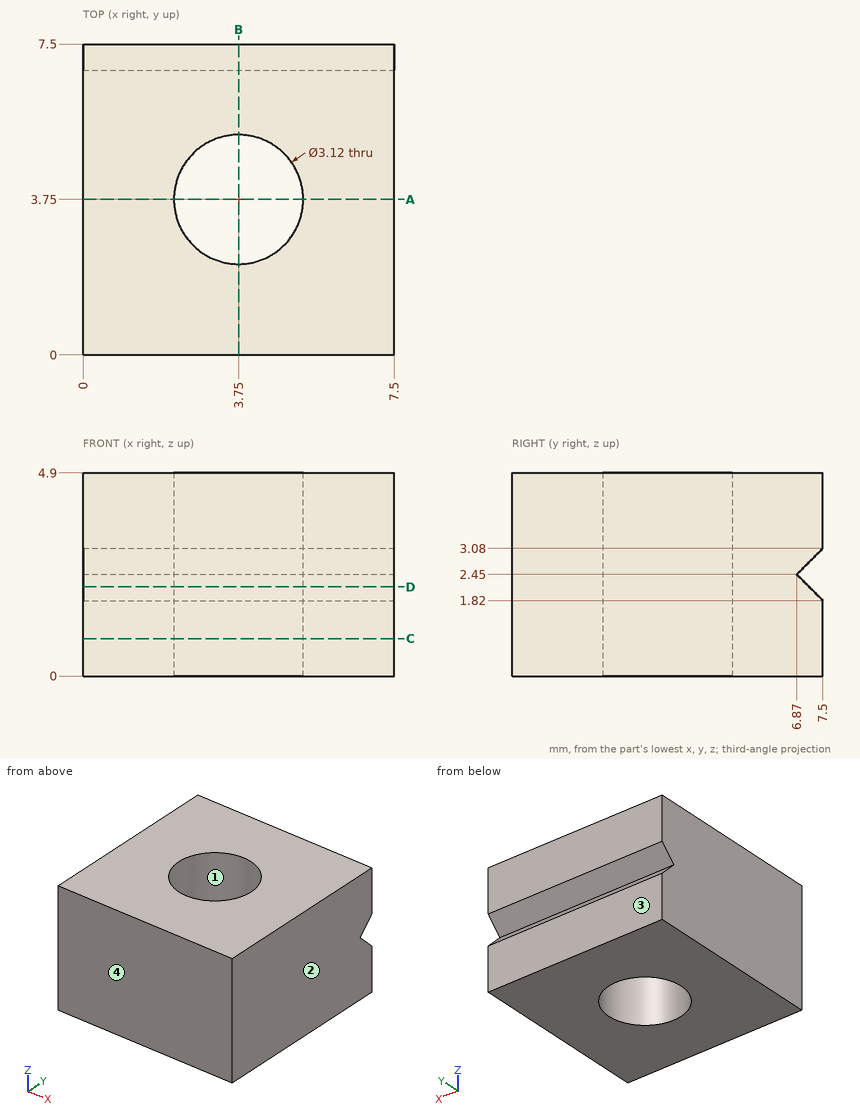
The figure shows three views and two pictorial views of one solid part (mm, origin at its lowest corner). Answer the questions. Coordinates: 2 decimals unless noted, no trailing zeros. Loops run counter-clockwise (first coordinate to the right, second up) from the corner with the lowest first, then second, coordinate; pieces in that order, holes last. Notation, with made-up numbers: (19.25, -8.5) -> (39.25, -8.5) arc R31 ccw to (39.25, 25.5) -> close; hole circle Ø2 at (63.5, 77.25). An arc over 180 degrees is marked (long way). Use one line per item in the form item = value. Start each with the question number.
Item 1: The part is cut by section C-C on z = 0.9. Determine the outline of the cut face in (x, y).
Item 2: The part is cut by section B-B on x = 3.75. Determine the outline of the cut face in (y, z).
Item 3: Consider L1, parallel to Y at x = 3.75, z = 1.3; L2, parallel to X at y = 3, z = 0.55; L3, parallel to Z at x = 4.25, y = 7.25. Determine where each line is inside the solid, lowest interval first. Write a range as [from, to].
Item 4: The part is cut by section D-D on z = 2.15. Determine the outline of the cut face in (x, y).
Item 5: The part is cut by section A-A on y = 3.75. Determine the outline of the cut face in (x, z).
Item 6: The mould has two halves that part along Y. Classify the marked faces 1, 2, 3 and 4: released by +Y, released by -Y, zero draft, split by the parting line, or undercut.
Answer key:
q1.outline = (0, 0) -> (7.5, 0) -> (7.5, 7.5) -> (0, 7.5) -> close; hole circle Ø3.12 at (3.75, 3.75)
q2.outline = (0, 0) -> (2.19, 0) -> (2.19, 4.9) -> (0, 4.9) -> close; (5.31, 0) -> (7.5, 0) -> (7.5, 1.82) -> (6.87, 2.45) -> (7.5, 3.08) -> (7.5, 4.9) -> (5.31, 4.9) -> close
q3.L1 = [0, 2.19], [5.31, 7.5]
q3.L2 = [0, 2.38], [5.12, 7.5]
q3.L3 = [0, 2.07], [2.83, 4.9]
q4.outline = (0, 0) -> (7.5, 0) -> (7.5, 7.17) -> (0, 7.17) -> close; hole circle Ø3.12 at (3.75, 3.75)
q5.outline = (0, 0) -> (2.19, 0) -> (2.19, 4.9) -> (0, 4.9) -> close; (5.31, 0) -> (7.5, 0) -> (7.5, 4.9) -> (5.31, 4.9) -> close
q6.face_1 = undercut
q6.face_2 = zero draft
q6.face_3 = released by +Y
q6.face_4 = released by -Y
